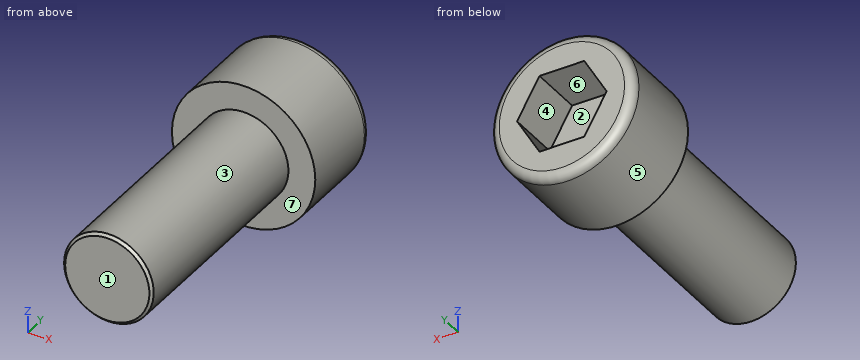
```python
from build123d import *

# Parameters (mm, degrees)
FILLET_1_R          = 1
CUT_EXTRUDE_START   = 10
CUT_EXTRUDE_1_DEPTH = 6
CHAMFER_1_SIZE      = 0.3


with BuildPart() as part:
    # 草图1 → 旋转1 (revolve)
    with BuildSketch(Plane.XY, mode=Mode.PRIVATE) as revolve_1_sk:
        Polygon((0, 10), (8, 10), (8, 0), (5, 0), (5, -25), (0, -25), align=None)
    revolve(revolve_1_sk.sketch.rotate(Axis((0, 10, 0), (0, -1, 0)), 180), axis=Axis((0, 10, 0), (0, -1, 0)))

    # 圆角1
    fillet_1_edges = [part.edges().sort_by_distance(p)[0] for p in [
        (8, 10, 0),
    ]]
    fillet(fillet_1_edges, radius=FILLET_1_R)

    # 草图2 → 切除-拉伸1 (cut)
    with BuildSketch(Plane(origin=(0, 0, 0), x_dir=(1, 0, 0), z_dir=(0, 1, 0)).offset(CUT_EXTRUDE_START)):
        Polygon((5, 0), (2.5, 4.330127019), (-2.5, 4.330127019), (-5, 0), (-2.5, -4.330127019), (2.5, -4.330127019), align=None)
    extrude(amount=-CUT_EXTRUDE_1_DEPTH, mode=Mode.SUBTRACT)

    # 倒角1
    chamfer_1_edges = [part.edges().sort_by_distance(p)[0] for p in [
        (5, -25, 0),
    ]]
    chamfer(chamfer_1_edges, length=CHAMFER_1_SIZE)


solid = part.part
```
Build history of the part. All positions in model axes, mm. Face numbers are marked on the shaded views. A direction names the side the tool comes from. Coordinates: 2 decimals unless noted, no trailing zeros. Order: outer loops, then holes, each group sorted by start corner. A loop starts at its lowest first (then second) coordinate and runs counter-clockwise, first axis right, second up. Notation, with made-up numbers: (77, 4.5) -> (94, 4.5) arc R25 ccw to (94, 35.5) -> close; hole circle Ø6 at (-24, -35). An arc over 180 degrees is marked (long way). Answer in a Markdown table with one row per item. Add a question column.
Q1. Band-saw the part on C-C, the plane y = -3.5. List the corners of the cut face in (x, z).
Q2. Band-saw the part on D-D, the plane y = 2.5. List the corners of the cut face in (x, z).
Q3. Mould opens along Z. For the marked faces 1, 2, 3 and 4 say: +Z half, -Z half, draft (parallel to the pull), parting line (faces both ways), or undercut.
Q4. Drop flat-ended pins along their axis: pin 1 (1 mm diameter, centred on y = 1.5, z = 3.5, fed in from +X); pin 2 (8 mm diameter, centred on x = -3, y = -9.5, fed in from -Z); pin 3 (1.5 mm diameter, centred on x = 1, y = 6.5, fed in from +Z). Give the stop position or say it passes through.
Q5. Which spindle directions (+Z, -Z, +X, -X, +Y, -Y) get a long thin tool onto all of the face, cutting with end or side? Do the marked faces 5, 6 and 7. Say none if no direction does.
Q6. Band-saw the part on B-B, the plane x = 0. List the corners of the cut face in (y, z), then the cut area to 3 significant figures.
Q7. Band-saw the part on A-A, the plane y = 7. List the corners of the cut face in (x, z), then the cut area to 3 significant figures.
Q8. Wall check: line 1 along Y through (x, z) = (1.75, -1.5); line 2 along Y through (x, z) = (1.75, -4.75); line 3 along X through (y, z) = (-20.5, -0.25). Give the ranges that are in metal, low to high. Write a range as [from, to].
Answers follow:
| question | item | result |
|---|---|---|
| 1 | outline | circle Ø10 at (0, 0) |
| 2 | outline | circle Ø16 at (0, 0) |
| 3 | face 1 | draft |
| 3 | face 2 | undercut |
| 3 | face 3 | parting line |
| 3 | face 4 | undercut |
| 4 | pin 1 | x = 7.42 |
| 4 | pin 2 | z = -5 |
| 4 | pin 3 | z = 8 |
| 5 | face 5 | +Y, -Y |
| 5 | face 6 | +Y |
| 5 | face 7 | -Y |
| 6 | outline | (-25, -4.7) -> (-24.7, -5) -> (0, -5) -> (0, -8) -> (9, -8) arc R1 ccw to (10, -7) -> (10, -4.33) -> (4, -4.33) -> (4, 4.33) -> (10, 4.33) -> (10, 7) arc R1 ccw to (9, 8) -> (0, 8) -> (0, 5) -> (-24.7, 5) -> (-25, 4.7) -> close |
| 6 | area | 358 mm^2 |
| 7 | outline | circle Ø16 at (0, 0); hole (-5, 0) -> (-2.5, -4.33) -> (2.5, -4.33) -> (5, 0) -> (2.5, 4.33) -> (-2.5, 4.33) -> close |
| 7 | area | 136 mm^2 |
| 8 | line 1 | [-25, 4] |
| 8 | line 2 | [0, 10] |
| 8 | line 3 | [-4.99, 4.99] |
